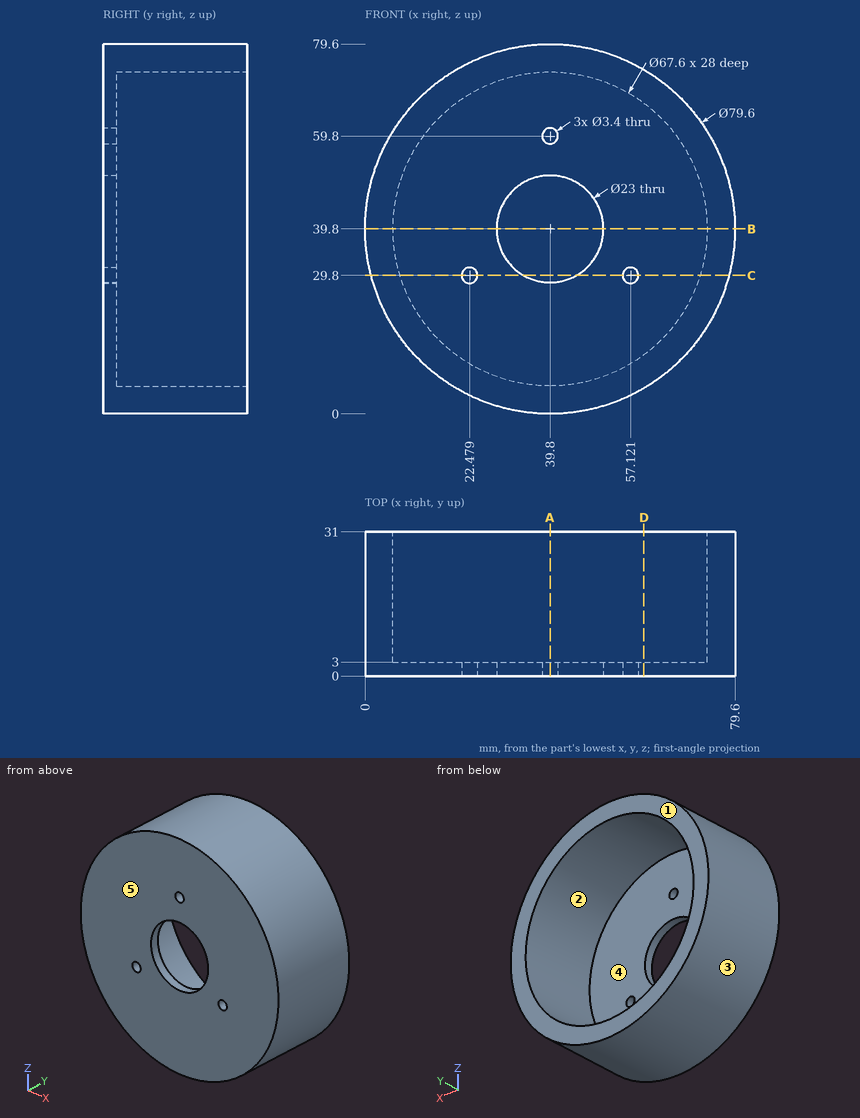
Could you check a few things on this drawing? It's one solid part, dimensions in mm from its lowest x, y, z. A direction names the side the tool comes from. Coordinates: 2 decimals unless noted, no trailing zeros. Order: outer loops, then holes, each group sorted by start corner. A loop starts at its lowest first (then second) coordinate and runs counter-clockwise, first axis right, second up.
1. I'm going to push flat-ended pins straight in: pin 1 (5 mm diameter, centred on x = 45.5, z = 16, fed in from +Y); pin 2 (3 mm diameter, centred on x = 64.5, y = 20, fed in from +Z); pin 3 (8 mm diameter, centred on x = 69.5, y = 11.5, fed in from -Z). Where does each tip first touch, or does it pass through?
2. If we section it at C-C (z = 29.8): Please give me the cut outline in (x, y), then the cut area to 3 significant figures.
3. If we section it at B-B (z = 39.8): Please give me the cut outline in (x, y), then the cut area to 3 significant figures.
4. If we section it at D-D (x = 60): Please give me the cut outline in (y, z).
5. Thinking about a two-plate mould opening in X: for the marked faces 3, 4 and 5, which applies, +X half, -X half, draft (parallel to the pull), parting line (faces both ways), or undercut?
6. I need wall thicknesses on line 1 (X direction, y = 11, z = 39); line 2 (Z direction, x = 39, y = 2); line 3 (X direction, y = 1.45, z = 39.8). Which ranges of each line are inside material? Lowest first, please.
7. If we section it at A-A (x = 39.8): Please give me the cut outline in (y, z).
8. For the marked faces 1 and 2, which set-ups out of +Z, -Z, +X, -X, +Y, -Y let a thin tool reach every point of the face, with its end or its side?
Entries:
1. pin 1: stops at y = 3
1. pin 2: stops at z = 72.14
1. pin 3: stops at z = 9.41
2. outline: (1.28, 0) - (20.78, 0) - (20.78, 3) - (7.51, 3) - (7.51, 31) - (1.28, 31) - close; (24.18, 0) - (34.12, 0) - (34.12, 3) - (24.18, 3) - close; (45.48, 0) - (55.42, 0) - (55.42, 3) - (45.48, 3) - close; (58.82, 0) - (78.32, 0) - (78.32, 31) - (72.09, 31) - (72.09, 3) - (58.82, 3) - close
2. area: 526 mm2
3. outline: (0, 0) - (28.3, 0) - (28.3, 3) - (6, 3) - (6, 31) - (0, 31) - close; (51.3, 0) - (79.6, 0) - (79.6, 31) - (73.6, 31) - (73.6, 3) - (51.3, 3) - close
3. area: 506 mm2
4. outline: (0, 5.51) - (31, 5.51) - (31, 12.7) - (3, 12.7) - (3, 66.9) - (31, 66.9) - (31, 74.09) - (0, 74.09) - close
5. face 3: parting line
5. face 4: undercut
5. face 5: draft
6. line 1: x = 0.01 to 6.01, 73.59 to 79.59
6. line 2: z = 0.01 to 28.33, 51.27 to 58.3, 61.3 to 79.59
6. line 3: x = 0 to 28.3, 51.3 to 79.6
7. outline: (0, 0) - (31, 0) - (31, 6) - (3, 6) - (3, 28.3) - (0, 28.3) - close; (0, 51.3) - (3, 51.3) - (3, 58.1) - (0, 58.1) - close; (0, 61.5) - (3, 61.5) - (3, 73.6) - (31, 73.6) - (31, 79.6) - (0, 79.6) - close
8. face 1: +Z, -Z, +X, -X, +Y
8. face 2: +Y
